Geometry: final body of the model. Coordinates: model frame, mm. A direction names the side the tool comes from. Give positions to 0.01 mm unless a question says otherwise; leave off trailing zeros. Loops run counter-clockwise (first coordinate to the right, second up) from the corner with the lowest first, then second, coordinate; pieces in that order, holes last. Notation, with made-up numbers: (44, -30) - (83, -30) arc R21 ccw to (83, -13) - close; hole circle Ø1 at (-12.5, -3). An arc over 180 degrees is marked (long way). Answer in a Markdown table with one row per item.
Autodesk Inventor part; units mm, degrees
ref_plane "YZ Plane" through (0, 0, 0) normal (1, 0, 0) x (0, 1, 0)
ref_plane "XZ Plane" through (0, 0, 0) normal (0, 1, 0) x (-1, 0, 0)
ref_plane "XY Plane" through (0, 0, 0) normal (0, 0, 1) x (1, 0, 0)
ref_plane "Plano de trabajo1" through (0, 27, 0) normal (0, 1, 0) x (1, 0, 0)
sketch "Boceto2" plane through (0, 27, 0) normal (0, 1, 0) x (1, 0, 0)
  line L0 (0, 10) -> (0, 15)
  line L1 (0, 15) -> (11.8906, 15)
  line L2 (0, 10) -> (0, 5)
  line L3 (0, 5) -> (15.0689, 5)
  line L4 (0, 5) -> (7, 5)
  line L5 (7, 5) -> (7, 15)
  line L6 (6.4875, 15) -> (4.4875, 15)
  circle A0 centre (4.4875, 15) radius 1.5
  circle A1 centre (4.4875, 5) radius 1.5
  line L7 (-42, 6) -> (-42, 0)
  line L8 (0, 0) -> (-42, 0)
  line L9 (-42, 0) -> (0, 0)
  line L10 (-21, 0) -> (-21, 36.5425)
  circle A2 centre (-46.4875, 15) radius 1.5
  circle A3 centre (-46.4875, 5) radius 1.5
  line L11 (0, 0) -> (1, 0)
  line L12 (1, 0) -> (8, 0)
  line L13 (8, 0) -> (8, 20)
  line L14 (8, 20) -> (1, 20)
  line L15 (1, 20) -> (1, 0)
  line L16 (-42, 10) -> (-42, 15)
  line L17 (-42, 15) -> (-53.8906, 15)
  line L18 (-42, 10) -> (-42, 5)
  line L19 (-42, 5) -> (-49, 5)
  line L20 (-49, 5) -> (-49, 15)
  line L21 (-48.4875, 15) -> (-46.4875, 15)
  circle A4 centre (-46.4875, 15) radius 1.5
  circle A5 centre (-46.4875, 5) radius 1.5
  line L22 (-42, 0) -> (-43, 0)
  line L23 (-43, 0) -> (-50, 0)
  line L24 (-50, 0) -> (-50, 20)
  line L25 (-50, 20) -> (-43, 20)
  line L26 (-43, 20) -> (-43, 0)
  line L27 (-43, 20) -> (-43, 21)
  line L28 (-43, 21) -> (1, 21)
  line L29 (1, 21) -> (1, 20)
  line L30 (-43, 0) -> (-43, -1)
  line L31 (-43, -1) -> (1, -1)
  line L32 (1, -1) -> (1, 0)
  line L33 (-50, 20) -> (-50, 24)
  line L34 (-50, 24) -> (8, 24)
  line L35 (-50, 0) -> (-50, -4)
  line L36 (-50, -4) -> (8, -4)
  line L37 (8, -4) -> (8, 0)
  line L38 (8, 24) -> (8, 19.2948)
  line L39 (-42, 10) -> (-42, 7)
  line L40 (-42, 7) -> (-58.0956, 7)
  line L41 (-51, 14) -> (-51, 6)
  line L42 (-42, 10) -> (-42, 13)
  line L43 (-42, 13) -> (-56.402, 13)
  point P0 (0, 20)
  point P1 (-42, 20)
  point P2 (-50, 13)
  point P3 (-43, 13)
  point P4 (-43, 7)
  point P5 (-50, 7)
  dimension "d8" = 5
  dimension "d9" = 5
  dimension "d10" = 7
  dimension "d11" = 2
  dimension "d12" = 3
  dimension "d13" = 3
  dimension "d14" = 1
  dimension "d15" = 7
  dimension "d16" = 1
  dimension "d17" = 1
  dimension "d18" = 4
  dimension "d19" = 4
  dimension "d22" = 3
  dimension "d23" = 3
extrude "Extrusión2" add sketch "Boceto2" along normal blind 4 contours L15 L14 L13 L1 A0 | L1 A0 L5 L3 A1 L15 | L3 A1 L13 L12 L15 | L29 L28 L10 L34 L38 L14 | L12 L37 L36 L35 L23 L30 L31 L32 | L28 L27 L25 L33 L34 L10 | L5 L1 L13 L3 | L23 L24 L40 L20 L19 A3 L26 | L26 L17 A2 L24 L25 | L19 A3 L20 L40 L26 | L26 L43 L20 L17 A2 | L17 L20 L43 L24
sketch "Boceto3" plane through (8, 27, -24) normal (0, 0, -1) x (-1, 0, 0)
  point P0 (8, -27)
sketch "Boceto4" plane through (8, 27, -24) normal (0, 0, -1) x (-1, 0, 0)
  line L0 (0, 4) -> (58, 4)
  line L1 (58, 4) -> (58, 18.1)
  line L2 (58, 18.1) -> (0, 18.1)
  line L3 (0, 18.1) -> (0, 4)
  line L4 (58, 18.1) -> (58, 22.1)
  line L5 (58, 18.1) -> (58, 32.1)
  line L6 (58, 32.1) -> (0, 32.1)
  line L7 (0, 32.1) -> (0, 18.1)
  line L8 (58, 18.1) -> (58, 28.6)
  line L9 (58, 28.6) -> (36.9156, 28.6)
  line L10 (8, -6.3468) -> (8, 18.1)
  line L11 (8, 18.1) -> (18.1, 18.1)
  line L12 (18.1, 18.1) -> (41.1, 18.1)
  line L13 (41.1, 18.1) -> (51.1, 18.1)
  line L14 (51.1, 18.1) -> (51.1, 26.6579)
  line L15 (51.1, 26.6579) -> (51.1, 31.1823)
  line L16 (51.1, 18.1) -> (51.1, 18)
  line L17 (51.1, 18.1) -> (51.2, 18.1)
  line L18 (51.2, 18.1) -> (51.2, 31.1)
  line L19 (51.2, 31.1) -> (41.1, 31.1)
  line L20 (41.1, 31.1) -> (41.1, 18.1)
  line L21 (51.2, 28.6) -> (49.2, 28.6)
  line L22 (41.1, 28.6) -> (43.1, 28.6)
  line L23 (43.1, 28.6) -> (43.15, 28.6)
  circle A0 centre (43.15, 28.6) radius 1.5
  line L24 (43.15, 28.6) -> (49.15, 28.6)
  circle A1 centre (49.15, 28.6) radius 1.5
  point P0 (8, -27)
  point P1 (8, 4)
  dimension "d24" = 14.1
  dimension "d25" = 4
  dimension "d26" = 14
  dimension "d27" = 10.5
  dimension "d28" = 10.1
  dimension "d29" = 23
  dimension "d30" = 10
  dimension "d31" = 0.1
  dimension "d32" = 0.1
  dimension "d33" = 13
  dimension "d34" = 10.1
  dimension "d35" = 2
  dimension "d36" = 2
  dimension "d38" = 0.05
  dimension "d39" = 3
  dimension "d40" = 6
  dimension "d41" = 3
extrude "Extrusión3" add sketch "Boceto4" along normal blind 5 contours L3 L2 L10 L0 | L10 L2 L1 L0 | L7 L6 L5 L9 L18 L19 L20 L2 | L2 L18 L9 L5 L4
sketch "Boceto5" plane through (8, 27, -29) normal (0, 0, -1) x (-1, 0, 0)
  line L0 (51.2, 18.1) -> (41.1, 18.1)
  line L1 (51.2, 18.1) -> (51.2, 28.6)
  line L2 (51.2, 31.1) -> (51.2, 18.1)
  line L3 (51.2, 28.6) -> (49.15, 28.6)
  circle A0 centre (49.15, 28.6) radius 1.5
  line L4 (49.15, 28.6) -> (43.15, 28.6)
  circle A1 centre (43.15, 28.6) radius 1.5
  line L5 (41.1, 18.1) -> (51.2, 18.1)
  line L6 (51.2, 18.1) -> (51.2, 31.1)
  line L7 (51.2, 31.1) -> (41.1, 31.1)
  line L8 (41.1, 31.1) -> (41.1, 18.1)
  point P0 (8, -27)
  dimension "d44" = 10.5
  dimension "d45" = 2.05
  dimension "d46" = 3
  dimension "d47" = 6
  dimension "d48" = 3
extrude "Extrusión4" add sketch "Boceto5" against normal blind 3
sketch "Boceto6" plane through (-50, 31, -24) normal (0, -1, 0) x (1, 0, 0)
  line L0 (58, -5) -> (0, -5)
  line L1 (0, 0) -> (58, 0)
  line L2 (58, 0) -> (58, -5)
  line L3 (58, -5) -> (0, -5)
  line L4 (0, -5) -> (0, 0)
  point P0 (50, 24)
extrude "Extrusión5" add sketch "Boceto6" along normal blind 4
sketch "Boceto7" plane through (8, 27, -24) normal (0, 0, 1) x (1, 0, 0)
  line L0 (-51.2, 31.1) -> (-72.2407, 31.1)
  line L1 (-51.2, 31.1) -> (-51.2, 18.1)
  line L2 (-51.2, 18.1) -> (-72.8631, 18.1)
  line L3 (-72.8631, 18.1) -> (-72.2407, 31.1)
  point P0 (-8, -27)
extrude "Extrusión6" cut sketch "Boceto7" against normal blind 2
sketch "Boceto8" plane through (-50, 27, -13) normal (-1, 0, 0) x (0, 0, 1)
  line L0 (-11, 31.1) -> (-11, 32.1)
  line L1 (-11, 32.1) -> (-11, 31.1)
  line L2 (-11, 31.1) -> (-13, 31.1)
  line L3 (-13, 18.1) -> (-13, 31.1)
  line L4 (-13, 31.1) -> (-13, 18.1)
  line L5 (-11, 18.1) -> (-13, 18.1)
  line L6 (-13, 18.1) -> (-11, 18.1)
  line L7 (-11, 18.1) -> (-11, 0.1456)
  line L8 (-11, 0.1456) -> (-11, 0)
  line L9 (0, 0) -> (-16, 0)
  line L10 (-16, 32.1) -> (-16, 0)
  line L11 (-11, 0) -> (-16, 0)
  line L12 (-16, 0) -> (-16, 32.1)
  line L13 (-11, 32.1) -> (-16, 32.1)
  line L14 (-16, 32.1) -> (-11, 32.1)
  point P0 (13, -27)
  point P1 (-13, 31.1)
extrude "Extrusión7" add sketch "Boceto8" along normal blind 19.1
sketch "Boceto10" plane through (8, 27, -24) normal (0, 0, 1) x (1, 0, 0)
  line L0 (-77.1, 18.1) -> (-73.389, 18.1)
  line L1 (-77.1, 18.1) -> (-41.1, 18.1)
  line L2 (-73.389, 18.1) -> (-73.389, 22.1)
  circle A0 centre (-73.389, 22.1) radius 1.5
  point P0 (-8, -27)
  dimension "d62" = 3.711
  dimension "d63" = 4
  dimension "d64" = 3
extrude "Extrusión9" cut sketch "Boceto10" against normal blind 19.1
sketch "Boceto11" plane through (8, 27, -24) normal (0, 0, 1) x (1, 0, 0)
  line L0 (-58, 0) -> (-77.1, 0)
  line L1 (-58, 0) -> (-77.1, 13.1321)
  line L2 (-77.1, 0) -> (-77.1, 18.1)
  line L3 (-58, 0) -> (-77.1, 0)
  line L4 (-77.1, 0) -> (-77.1, 13.1321)
  line L5 (-61.7227, 0) -> (-77.1, 13.1321)
  line L6 (-61.7227, 0) -> (-77.1, 0)
  point P0 (-8, -27)
extrude "Extrusión10" cut sketch "Boceto11" against normal blind 19.1 contours L0 L2 L5
fillet "Empalme1" radius 15 1 edges at (8, 59.1, -26.5)
chamfer "Chaflán1" distance 1 angle 45 2 edges at (-51.1, 45.1, -24) (-33.1, 51.6, -24)
properties part number "servov2"
Q1. Draft query along Y for faces 4 (the flat face through (-50, 29, -2)), 5 (the cylindrical face through (-41.956, 56.865, -27.521)), 6 (the flat face through (-38, 59.1, -26)). Return one class per face: pulls with the +Y half, pulls with the -Y half, needs draft (parallel to the pull), parting line crosses it, or undercut.
Check values:
| item | result |
|---|---|
| face 4 | needs draft |
| face 5 | undercut |
| face 6 | pulls with the +Y half |
Q2. Cut plane A-A (z = -5). Output: boundary loops of the cut face in (x, y).
Check values:
| item | result |
|---|---|
| outline | (-50, 27) - (-47.99, 27) - (-47.99, 31) - (-50, 31) - close; (-44.99, 27) - (-43, 27) - (-43, 31) - (-44.99, 31) - close; (1, 27) - (2.99, 27) - (2.99, 31) - (1, 31) - close; (5.99, 27) - (8, 27) - (8, 31) - (5.99, 31) - close |
Q3. First-contact query: pin 1 (4 mm diameter, centred on x = -26.5, y = 35.5, fed in from +Z); pin 2 (3.5 mm diameter, centred on x = -65.389, y = 49.1, fed in from +Z); pin 3 (1.8 mm diameter, centred on x = -46.49, z = -5, fed in from +Y); pin 4 (2 mm diameter, centred on y = 28.5, z = -12.5, fed in from -X). Flat tips, straight axial feed; report the tip coordinate or a pass-through.
Check values:
| item | result |
|---|---|
| pin 1 | z = -24 |
| pin 2 | z = -26 |
| pin 3 | through |
| pin 4 | x = -50 |
Q4. Cut plane D-D (x = -35.15). Output: boundary loops of the cut face in (y, z), and give its area (3 significant figures).
Check values:
| item | result |
|---|---|
| outline | (27, -29) - (54.1, -29) - (54.1, -26) - (45.1, -26) - (45.1, -25) - (44.1, -24) - (31, -24) - (31, -21) - (27, -21) - close; (27, 1) - (31, 1) - (31, 4) - (27, 4) - close; (57.1, -29) - (59.1, -29) - (59.1, -24) - (58.1, -24) - (58.1, -26) - (57.1, -26) - close |
| area | 149 mm² |
Q5. Cut plane B-B (x = -12). Output: boundary loops of the cut face in (y, z), and give its area (4 significant figures).
Check values:
| item | result |
|---|---|
| outline | (27, -29) - (59.1, -29) - (59.1, -24) - (31, -24) - (31, -21) - (27, -21) - close; (27, 1) - (31, 1) - (31, 4) - (27, 4) - close |
| area | 184.5 mm² |
Q6. Reachability of faces 1 (the flat face through (-46, 29, -7)), 2 (the flat face through (-43, 29, -3)), 3 (the flat face through (-51, 52, -26)) from +Z, -Z, +X, -X, +Y, -Y: full face, straight path, thin tool, end or side. Return the list, or none.
Check values:
| item | result |
|---|---|
| face 1 | -X, +Y, -Y |
| face 2 | +Y, -Y |
| face 3 | +Z, -X |
Q7. Cut plane C-C (z = -20). Output: boundary loops of the cut face in (x, y).
Check values:
| item | result |
|---|---|
| outline | (-50, 27) - (-43, 27) - (-43, 31) - (-50, 31) - close; (1, 27) - (8, 27) - (8, 31) - (1, 31) - close |
Q8. Material intervals for line 1 along X through (y, z) = (28.4, -15); line 2 along Y through (x, z) = (-41.15, -27.75); line 3 along Z through (x, y) = (-46, 49.5), sorted ascending.
Check values:
| item | result |
|---|---|
| line 1 | -50 to -47.99, -44.99 to -43, 1 to 2.99, 5.99 to 8 |
| line 2 | 27 to 54.1, 57.1 to 59.1 |
| line 3 | -29 to -26 |
